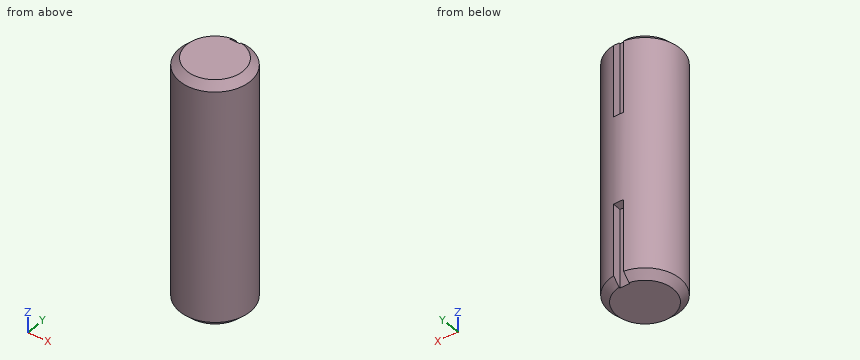
from build123d import *

# Parameters (mm, degrees)
SKETCH1_R      = 12.7
EXTRUDE1_DEPTH = 88.9
SKETCH2_W      = 3.556
SKETCH2_H      = 3.175
EXTRUDE2_DEPTH = 28.575
CHAMFER1_SIZE  = 2.54
CHAMFER2_SIZE  = 2.54


with BuildPart() as part:
    # Sketch1 → Extrude1 (new body)
    with BuildSketch(Plane.XY):
        Circle(SKETCH1_R)
    extrude(amount=-EXTRUDE1_DEPTH)

    # Sketch2 → Extrude2 (cut)
    with BuildSketch(Plane.XY):
        with Locations((0, 11.1125)):
            Rectangle(SKETCH2_W, SKETCH2_H)
    extrude2 = extrude(amount=-EXTRUDE2_DEPTH, mode=Mode.SUBTRACT)

    # Chamfer1
    chamfer1_edges = [part.edges().sort_by_distance(p)[0] for p in [
        (-8.327946926, -9.588289733, 0),
    ]]
    chamfer(chamfer1_edges, length=CHAMFER1_SIZE)

    # Mirror5: Extrude2 across plane
    add(extrude2.mirror(Plane.XY.offset(-44.45)), mode=Mode.SUBTRACT)

    # Chamfer2
    chamfer2_edges = [part.edges().sort_by_distance(p)[0] for p in [
        (-8.327946926, -9.588289733, -88.9),
    ]]
    chamfer(chamfer2_edges, length=CHAMFER2_SIZE)


solid = part.part
Can you work these out from the model? Positions are in its coordinate system, mm. Round coordinates to 2 decimals unless told otherwise and drop trailing zeros. Order: outer loops, then holes, each group sorted by start corner. A loop starts at its lowest first (then second) coordinate and runs counter-clockwise, first axis right, second up. Notation, with made-up numbers: (85, -32) - (112, -32) arc R15 cw to (112, -8) - close; hole circle Ø3 at (37, 18.25). An arc over 180 degrees is marked (long way). Answer in a Markdown table with one row per item.
(1) Suppose I cut it at A-A, the plane x = 0. Please give me the cut outline in (y, z) (3 decimals), plus the area to 3 significant figures.
From the geometry:
| item | result |
|---|---|
| outline | (-12.7, -86.36) - (-10.16, -88.9) - (9.525, -88.9) - (9.525, -60.325) - (12.7, -60.325) - (12.7, -28.575) - (9.525, -28.575) - (9.525, 0) - (-10.16, 0) - (-12.7, -2.54) - close |
| area | 2,070 mm2 |
(2) Suppose I cut it at B-B, the plane z = -49. Please give me the cut outline in (x, y), plus the area to 3 significant figures.
From the geometry:
| item | result |
|---|---|
| outline | circle Ø25.4 at (0, 0) |
| area | 507 mm2 |
(3) Please list where these lines run through material, in increasing order: L1, parallel to X at y = -0.25, z = -19; L2, parallel to X at y = 4.5, z = -65; L3, parallel to Z at x = -4.5, y = -9.75. Write a range as from..to.
From the geometry:
| item | result |
|---|---|
| L1 | x = -12.7..12.7 |
| L2 | x = -11.88..11.88 |
| L3 | z = -88.32..-0.58 |
(4) For P1, Ø2.5, axis at y = 11, z = -76, coming from the +X side; P2, Ø1.1, axis at x = 0, z = -11.5, coming from the +Y side (3 decimals); P3, Ø2.5, axis at y = 11.5, z = -69.5, coming from the -X side; P4, Ø1, axis at x = 3, y = -7.5, coming from the +Z side, each with a flat end and sliding along its axis, tell me the tip position at first contact or that it passes through.
From the geometry:
| item | result |
|---|---|
| P1 | stops at x = 8.14 |
| P2 | stops at y = 9.525 |
| P3 | stops at x = -7.5 |
| P4 | stops at z = 0 |
